Build history of the part. All positions in model axes, mm. A direction names the side the tool comes from. Round coordinates to 2 decimals unless told otherwise and drop trailing zeros. Order: outer loops, then holes, each group sorted by start corner. A loop starts at its lowest first (then second) coordinate and runs counter-clockwise, first axis right, second up. Notation, with made-up numbers: (41.5, 43) -> (58.5, 43) arc R21 cw to (58.5, 72) -> close; hole circle Ø9 at (64, 29.5). An arc over 180 degrees is marked (long way). Use a Markdown table: item, result. Add a question column.
Item 1: 3-axis set-ups, long thin cutter, end or side, ignore diameter. For faces 4 (the face through (14, -197, 3.175)), 5 (the face through (13, -197, 0)): which of +Z, -Z, +X, -X, +Y, -Y reach the whole face in a straight line?
Item 2: Slice it at B-B, the plane z = 12.7. Give the cut face in (x, y) (3 decimals).
Item 3: Probe L1, parallel to Z at x = 12.7, y = -2.3; L2, parallel to Y at x = 23.25, z = 21.75 (3 decimals); L3, parallel to Z at x = 7.75, y = -100.5 (3 decimals). List the from-to ranges inside material, lowest first.
Item 4: Slice it at A-A, the plane x = 12.7. Give the cut face in (y, z) (3 decimals), plus the area to 3 significant figures.
Item 5: Two-plate mould, pull along Y, no slides. Class faces 1 (the face through (3.175, -197, 14)), 2 (the face through (10, 0, 10)), 3 (the face through (25.4, -199, 1)): released by +Y, released by -Y, zero draft, split by the parting line, or undercut.
Item 6: Pin check, flat tips, straight feed: pin 1 (6.5 mm diameter, centred on y = -134.5, z = 11, fed in from +X) (3 decimals); pin 2 (6.5 mm diameter, centred on x = 15.5, y = -102, fed in from +Z) (3 decimals). Stop position of each tip, or through.
Item 7: Slice it at C-C, the plane y = -294. Give the cut face in (x, z) (3 decimals).
from build123d import *

# Parameters (mm, degrees)
F1_DEPTH = 400.05
F2_W     = 22.225
F2_H     = 22.225
F3_DEPTH = 3.175
F4_W     = 22.225
F4_H     = 22.225
F5_DEPTH = 3.175
F7_D     = 6.7564


with BuildPart() as f1:
    # F0 (on Front) → F1 (new body)
    with BuildSketch(Plane.XZ):
        Polygon((0, 25.4), (0, 0), (25.4, 0), (25.4, 3.175), (3.175, 3.175), (3.175, 25.4), align=None)
    extrude(amount=F1_DEPTH)

    # F2 (on face) → F3 (join)
    with BuildSketch(Plane.XZ.offset(400.05)):
        with Locations((14.2875, 14.2875)):
            Rectangle(F2_W, F2_H)
    extrude(amount=-F3_DEPTH)

    # F4 (on face) → F5 (join)
    with BuildSketch(Plane(origin=(0, 0, 0), x_dir=(-1, 0, 0), z_dir=(0, 1, 0))):
        with Locations((-14.2875, 14.2875)):
            Rectangle(F4_W, F4_H)
    extrude(amount=-F5_DEPTH)

    # F7 (through all)
    with Locations(Plane.XZ.offset(400.05)):
        with Locations((12.7, 12.7)):
            Hole(F7_D / 2)


solid = f1.part
Check sheet entries:
| question | item | result |
|---|---|---|
| 1 | face 4 | +Z, +X |
| 1 | face 5 | -Z, +X, -X, +Y, -Y |
| 2 | outline | (0, -400.05) -> (9.322, -400.05) -> (9.322, -396.875) -> (3.175, -396.875) -> (3.175, -3.175) -> (9.322, -3.175) -> (9.322, 0) -> (0, 0) -> close; (16.078, -400.05) -> (25.4, -400.05) -> (25.4, -396.875) -> (16.078, -396.875) -> close; (16.078, -3.175) -> (25.4, -3.175) -> (25.4, 0) -> (16.078, 0) -> close |
| 3 | L1 | 0 to 9.32, 16.08 to 25.4 |
| 3 | L2 | -400.05 to -396.875, -3.175 to 0 |
| 3 | L3 | 0 to 3.175 |
| 4 | outline | (-400.05, 0) -> (0, 0) -> (0, 9.322) -> (-3.175, 9.322) -> (-3.175, 3.175) -> (-396.875, 3.175) -> (-396.875, 9.322) -> (-400.05, 9.322) -> close; (-400.05, 16.078) -> (-396.875, 16.078) -> (-396.875, 25.4) -> (-400.05, 25.4) -> close; (-3.175, 16.078) -> (0, 16.078) -> (0, 25.4) -> (-3.175, 25.4) -> close |
| 4 | area | 1,370 mm2 |
| 5 | face 1 | undercut |
| 5 | face 2 | released by +Y |
| 5 | face 3 | zero draft |
| 6 | pin 1 | x = 3.175 |
| 6 | pin 2 | z = 3.175 |
| 7 | outline | (0, 0) -> (25.4, 0) -> (25.4, 3.175) -> (3.175, 3.175) -> (3.175, 25.4) -> (0, 25.4) -> close |
